Geometry check sheet. Reference: the model listing, model coordinates, mm. Coordinates: 2 decimals unless noted, no trailing zeros. Write each loop counter-clockwise with the first axis right and the second up, starting at its lowest first coordinate (ties: lowest second). Pieces come first, ordered by that corner, then holes.
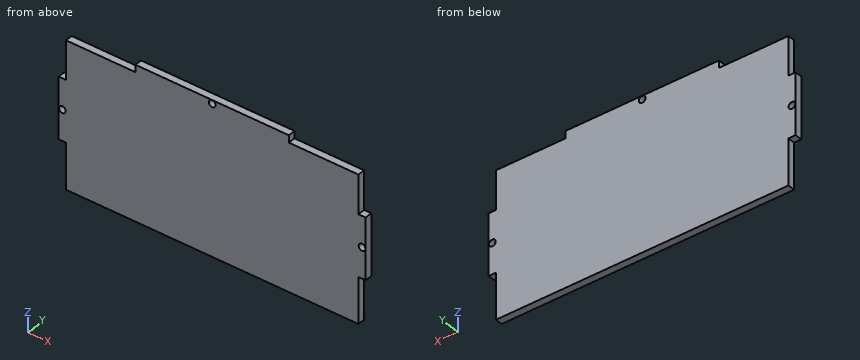
from build123d import *

# Parameters (mm, degrees)
SKETCH1_W           = 127
SKETCH1_H           = 63.5
BOSS_EXTRUDE1_DEPTH = 2.9972
CUT_EXTRUDE1_REACH  = 73.058
SKETCH2_R           = 1.397
SKETCH2_W           = 2.9972
SKETCH2_H           = 19.05


with BuildPart() as part:
    # Sketch1 → Boss-Extrude1 (new body)
    with BuildSketch(Plane(origin=(0, 0, 0), x_dir=(1, 0, 0), z_dir=(0, 1, 0))):
        Rectangle(SKETCH1_W, SKETCH1_H)
    extrude(amount=BOSS_EXTRUDE1_DEPTH)

    # Sketch2 → Cut-Extrude1 (cut, up to next)
    with BuildSketch(Plane(origin=(0, 2.9972, 0), x_dir=(1, 0, 0), z_dir=(0, 1, 0)), mode=Mode.PRIVATE) as cut_extrude1_sk1:
        with Locations(Location((0, -30.2514, 0), (0, 0, 90))):
            Circle(SKETCH2_R)
    cut_extrude1_tool1 = extrude(cut_extrude1_sk1.sketch, amount=-CUT_EXTRUDE1_REACH, mode=Mode.PRIVATE) & part.part
    # Sketch2 → Cut-Extrude1 (cut, up to next)
    with BuildSketch(Plane(origin=(0, 2.9972, 0), x_dir=(1, 0, 0), z_dir=(0, 1, 0)), mode=Mode.PRIVATE) as cut_extrude1_sk2:
        with Locations(Location((-62.0014, 0, 0), (0, 0, 270))):
            Circle(SKETCH2_R)
    cut_extrude1_tool2 = extrude(cut_extrude1_sk2.sketch, amount=-CUT_EXTRUDE1_REACH, mode=Mode.PRIVATE) & part.part
    # Sketch2 → Cut-Extrude1 (cut, up to next)
    with BuildSketch(Plane(origin=(0, 2.9972, 0), x_dir=(1, 0, 0), z_dir=(0, 1, 0)), mode=Mode.PRIVATE) as cut_extrude1_sk3:
        with Locations(Location((62.0014, 0, 0), (0, 0, 90))):
            Circle(SKETCH2_R)
    cut_extrude1_tool3 = extrude(cut_extrude1_sk3.sketch, amount=-CUT_EXTRUDE1_REACH, mode=Mode.PRIVATE) & part.part
    # Sketch2 → Cut-Extrude1 (cut, up to next)
    with BuildSketch(Plane(origin=(0, 2.9972, 0), x_dir=(1, 0, 0), z_dir=(0, 1, 0)), mode=Mode.PRIVATE) as cut_extrude1_sk4:
        Polygon((63.5, -31.75), (31.75, -31.75), (31.75, -28.7528), (60.5028, -28.7528), (60.5028, -12.7), (63.5, -12.7), (63.5, -28.7528), align=None)
    cut_extrude1_tool4 = extrude(cut_extrude1_sk4.sketch, amount=-CUT_EXTRUDE1_REACH, mode=Mode.PRIVATE) & part.part
    # Sketch2 → Cut-Extrude1 (cut, up to next)
    with BuildSketch(Plane(origin=(0, 2.9972, 0), x_dir=(1, 0, 0), z_dir=(0, 1, 0)), mode=Mode.PRIVATE) as cut_extrude1_sk5:
        with Locations((-62.0014, 22.225)):
            Rectangle(SKETCH2_W, SKETCH2_H)
    cut_extrude1_tool5 = extrude(cut_extrude1_sk5.sketch, amount=-CUT_EXTRUDE1_REACH, mode=Mode.PRIVATE) & part.part
    # Sketch2 → Cut-Extrude1 (cut, up to next)
    with BuildSketch(Plane(origin=(0, 2.9972, 0), x_dir=(1, 0, 0), z_dir=(0, 1, 0)), mode=Mode.PRIVATE) as cut_extrude1_sk6:
        Polygon((-63.5, -31.75), (-31.75, -31.75), (-31.75, -28.7528), (-60.5028, -28.7528), (-60.5028, -12.7), (-63.5, -12.7), (-63.5, -28.7528), align=None)
    cut_extrude1_tool6 = extrude(cut_extrude1_sk6.sketch, amount=-CUT_EXTRUDE1_REACH, mode=Mode.PRIVATE) & part.part
    # Sketch2 → Cut-Extrude1 (cut, up to next)
    with BuildSketch(Plane(origin=(0, 2.9972, 0), x_dir=(1, 0, 0), z_dir=(0, 1, 0)), mode=Mode.PRIVATE) as cut_extrude1_sk7:
        with Locations((62.0014, 22.225)):
            Rectangle(SKETCH2_W, SKETCH2_H)
    cut_extrude1_tool7 = extrude(cut_extrude1_sk7.sketch, amount=-CUT_EXTRUDE1_REACH, mode=Mode.PRIVATE) & part.part
    add(cut_extrude1_tool1.solids().sort_by_distance((0, 2.9972, 30.2514))[0], mode=Mode.SUBTRACT)
    add(cut_extrude1_tool2.solids().sort_by_distance((-62.0014, 2.9972, 0))[0], mode=Mode.SUBTRACT)
    add(cut_extrude1_tool3.solids().sort_by_distance((62.0014, 2.9972, 0))[0], mode=Mode.SUBTRACT)
    add(cut_extrude1_tool4.solids().sort_by_distance((47.625, 2.9972, 31.379735))[0], mode=Mode.SUBTRACT)
    add(cut_extrude1_tool5.solids().sort_by_distance((-62.0014, 2.9972, -22.225))[0], mode=Mode.SUBTRACT)
    add(cut_extrude1_tool6.solids().sort_by_distance((-47.625, 2.9972, 31.379735))[0], mode=Mode.SUBTRACT)
    add(cut_extrude1_tool7.solids().sort_by_distance((62.0014, 2.9972, -22.225))[0], mode=Mode.SUBTRACT)


solid = part.part
1. Sectioned sample at D-D, the plane z = -28. Record the boundary of the cut face in (x, y), and give its area (3 significant figures).
Computed values:
outline: (-60.5, 0) - (60.5, 0) - (60.5, 3) - (-60.5, 3) - close
area: 363 mm2
2. Thickness scan on line 1 along X through (y, z) = (2.6, 26.5); line 2 along Z through (x, y) = (-42.5, 1.3). Record the ranges inside material, lowest first.
Computed values:
line 1: x = -60.5 to 60.5
line 2: z = -31.75 to 28.75
3. Sectioned sample at C-C, the plane x = 51.5. Record the boundary of the cut face in (y, z), and give its area (3 significant figures).
Computed values:
outline: (0, -31.75) - (3, -31.75) - (3, 28.75) - (0, 28.75) - close
area: 181 mm2
4. Gauge pin test, flat ends, axial feed: pin 1 Ø3.5 at (x, z) = (62, 0) entering from -Y; pin 2 Ø1.5 at (x, y) = (61.5, 2) entering from -Z; pin 3 Ø0.9 at (y, z) = (2, 23.5) entering from +X; pin 4 Ø1.5 at (y, z) = (2, 23.5) entering from -X. Record the tip position at first contact, or that the pin passes through.
Computed values:
pin 1: stops at y = 0
pin 2: stops at z = -12.7
pin 3: stops at x = 60.5
pin 4: stops at x = -60.5
5. Sectioned sample at B-B, the plane z = 0. Record the boundary of the cut face in (x, y), and give its area (3 significant figures).
Computed values:
outline: (-63.5, 0) - (-63.4, 0) - (-63.4, 3) - (-63.5, 3) - close; (-60.6, 0) - (60.6, 0) - (60.6, 3) - (-60.6, 3) - close; (63.4, 0) - (63.5, 0) - (63.5, 3) - (63.4, 3) - close
area: 364 mm2
6. Sectioned sample at A-A, the plane x = 0. Record the boundary of the cut face in (y, z), and give its area (3 significant figures).
Computed values:
outline: (0, -31.75) - (3, -31.75) - (3, 28.85) - (0, 28.85) - close; (0, 31.65) - (3, 31.65) - (3, 31.75) - (0, 31.75) - close
area: 182 mm2
